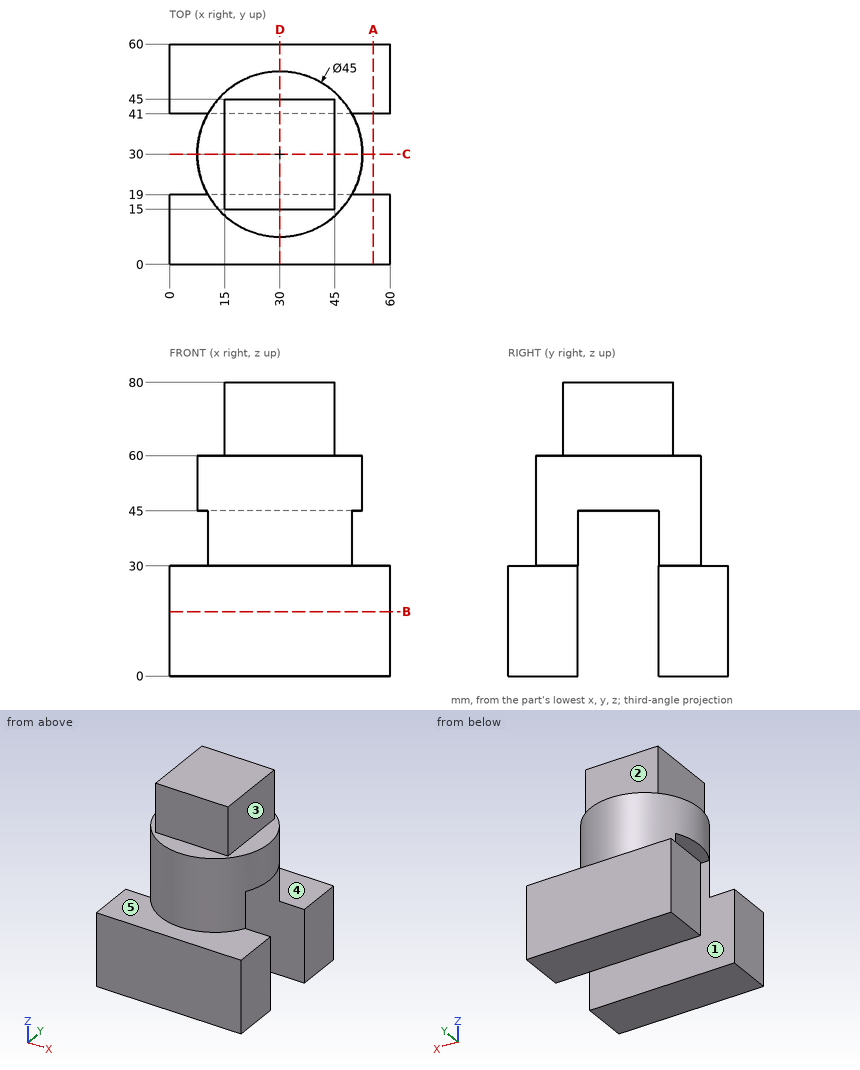
Job drawing, mm, ordinate dimensions from the low corner. One solid piece. A direction names the side the tool comes from. Round coordinates to 2 decimals unless told otherwise and drop trailing zeros. Loops run counter-clockwise (first coordinate to the right, second up) from the corner with the lowest first, then second, coordinate; pieces in that order, holes last. Notation, with made-up numbers: (4.5, -3) -> (36.5, -3) arc R19 ccw to (36.5, 24) -> close; hole circle Ø10 at (59, -31). An arc over 180 degrees is marked (long way). Use a Markdown table: item, result.
1) Cut at A-A, the plane x = 55.5. List the corners of the cut face in (y, z).
The answers:
| item | result |
|---|---|
| outline | (0, 0) -> (19, 0) -> (19, 30) -> (0, 30) -> close; (41, 0) -> (60, 0) -> (60, 30) -> (41, 30) -> close |
2) Tool access for the marked faces 1, 2, 3, 4 and 5: list every direction of +Z, -Z, +X, -X, +Y, -Y with a clear straight run to the whole face (end or side of a thin tool).
The answers:
| item | result |
|---|---|
| face 1 | -Z, +X, -X |
| face 2 | +Z, +X, -X, +Y |
| face 3 | +Z, +X, +Y, -Y |
| face 4 | +Z, +Y |
| face 5 | +Z, -Y |
3) Probe line 1 (Y direction, x = 49.5, z = 7.5); line 2 (Z direction, x = 27, y = 53.5); line 3 (Z direction, x = 48.5, y = 39.5). List the from-to ranges inside material, lowest first. Write a range as [from, to].
The answers:
| item | result |
|---|---|
| line 1 | y = [0, 19], [41, 60] |
| line 2 | z = [0, 30] |
| line 3 | z = [45, 60] |
4) Cut at B-B, the plane z = 17.5. List the corners of the cut face in (x, y), and give its area (3 significant figures).
The answers:
| item | result |
|---|---|
| outline | (0, 0) -> (60, 0) -> (60, 19) -> (0, 19) -> close; (0, 41) -> (60, 41) -> (60, 60) -> (0, 60) -> close |
| area | 2,280 mm2 |
5) Cut at D-D, the plane x = 30. List the corners of the cut face in (y, z), and give its area (3 significant figures).
The answers:
| item | result |
|---|---|
| outline | (0, 0) -> (19, 0) -> (19, 45) -> (41, 45) -> (41, 0) -> (60, 0) -> (60, 30) -> (52.5, 30) -> (52.5, 60) -> (45, 60) -> (45, 80) -> (15, 80) -> (15, 60) -> (7.5, 60) -> (7.5, 30) -> (0, 30) -> close |
| area | 2,760 mm2 |
6) Cut at C-C, the plane y = 30. List the corners of the cut face in (x, z), and give its area (4 significant figures).
The answers:
| item | result |
|---|---|
| outline | (7.5, 45) -> (52.5, 45) -> (52.5, 60) -> (45, 60) -> (45, 80) -> (15, 80) -> (15, 60) -> (7.5, 60) -> close |
| area | 1,275 mm2 |
7) Drop flat-ended pins along their axis: pin 1 Ø8 at (x, z) = (20.5, 60) entering from -Y; pin 2 Ø4 at (x, y) = (16, 53) entering from -Z; pin 3 Ø6 at (x, z) = (30, 67.5) entering from -Y; pin 4 Ø12 at (x, z) = (29.5, 45.5) entering from -Y. Give the stop position or say it passes through.
The answers:
| item | result |
|---|---|
| pin 1 | stops at y = 8.18 |
| pin 2 | stops at z = 0 |
| pin 3 | stops at y = 15 |
| pin 4 | stops at y = 7.5 |
